Design review of the part built by this model. Coordinates are the model's own, in mm. A direction names the side the tool comes from. Give positions to 0.01 mm unless a question says otherwise; leave off trailing zeros. Write each loop counter-clockwise with the first axis right and the second up, starting at its lowest first coordinate (ties: lowest second). Pieces come first, ordered by that corner, then holes. Notation, with made-up numbers: (88, 23) -> (100, 23) arc R16 ccw to (100, 42) -> close; hole circle Ø4 at (33, 35). An arc over 180 degrees is marked (long way). Use CSV: the item, a comma, the result in double quotes.
```python
from build123d import *

# Parameters (mm, degrees)
SKETCH_1_W               = 60
SKETCH_1_H               = 10
EXTRUDE_1_DEPTH          = 8
SKETCH_2_W               = 10
SKETCH_2_H               = 21
SKETCH_2_R               = 3
EXTRUDE_2_DEPTH          = 5
FILLET_1_R               = 3
SKETCH_3_R               = 1.1
EXTRUDE_3_DEPTH          = 4
SKETCH_5_W               = 10
SKETCH_5_H               = 2
EXTRUDE_4_DEPTH          = 10
FILLET_4_R               = 1
SKETCH_4_R               = 1.6
CUT_EXTRUDE_1_DEPTH      = 17.792928464
CUT_EXTRUDE_1_DEPTH_BACK = 16.892331711


with BuildPart() as part:
    # 草图1 → 凸台-拉伸1 (new body)
    with BuildSketch(Plane(origin=(0, 0, 0), x_dir=(1, 0, 0), z_dir=(0, 1, 0))):
        Rectangle(SKETCH_1_W, SKETCH_1_H)
    extrude(amount=EXTRUDE_1_DEPTH)

    # 草图2 → 凸台-拉伸2 (add)
    with BuildSketch(Plane(origin=(30, 0, 0), x_dir=(0, 0, -1), z_dir=(1, 0, 0))):
        with Locations((0, -2.5)):
            Rectangle(SKETCH_2_W, SKETCH_2_H)
        with Locations((0, -8)):
            Circle(SKETCH_2_R, mode=Mode.SUBTRACT)
    extrude_2 = extrude(amount=-EXTRUDE_2_DEPTH)

    # 镜向1: 凸台-拉伸2 across plane
    add(extrude_2.mirror(Plane(origin=(0, 0, 0), x_dir=(0, 0, 1), z_dir=(1, 0, 0))))

    # 圆角1
    fillet_1_edges = [part.edges().sort_by_distance(p)[0] for p in [
        (27.5, -13, 5),
        (27.5, -13, -5),
        (-27.5, -13, -5),
        (-27.5, -13, 5),
    ]]
    fillet(fillet_1_edges, radius=FILLET_1_R)

    # 草图3 → 凸台-拉伸3 (add)
    with BuildSketch(Plane.ZY.offset(-5)):
        Polygon((-6.5, -2), (17.5, -2), (17.5, -8), (17.5, -10.376383694), (21.792928464, -10.376383694), (21.792928464, 2.519827065), (-10.892331711, 2.519827065), (-10.892331711, -10.376383694), (-6.5, -10.376383694), (-6.5, -8), align=None)
        with Locations((-8.5, -8)):
            Circle(SKETCH_3_R, mode=Mode.SUBTRACT)
        with Locations((19.5, -8)):
            Circle(SKETCH_3_R, mode=Mode.SUBTRACT)
    extrude(amount=-EXTRUDE_3_DEPTH)

    # 草图5 → 凸台-拉伸4 (add)
    with BuildSketch(Plane.ZY.offset(-5)):
        with Locations((0, -1)):
            Rectangle(SKETCH_5_W, SKETCH_5_H)
    extrude(amount=EXTRUDE_4_DEPTH)

    # 圆角4
    fillet_4_edges = [part.edges().sort_by_distance(p)[0] for p in [
        (5, 0.259913532, -5),
        (7, 2.519827065, -5),
        (9, 1.259913532, -5),
        (7, 2.519827065, -10.892331711),
        (5, 0.259913532, 5),
        (7, -10.376383694, -10.892331711),
        (7, 2.519827065, 5),
        (7, 2.519827065, 21.792928464),
        (7, -10.376383694, 21.792928464),
        (9, 1.259913532, 5),
        (9, 0, 0),
    ]]
    fillet(fillet_4_edges, radius=FILLET_4_R)

    # 草图4 → 切除-拉伸1 (cut, two sides)
    with BuildSketch(Plane.XY.offset(5)) as cut_extrude_1_sk:
        with Locations((-15, 4)):
            Circle(SKETCH_4_R)
        with Locations((15, 4)):
            Circle(SKETCH_4_R)
    extrude(amount=CUT_EXTRUDE_1_DEPTH, mode=Mode.SUBTRACT)
    extrude(cut_extrude_1_sk.sketch, amount=-CUT_EXTRUDE_1_DEPTH_BACK, mode=Mode.SUBTRACT)


solid = part.part
```
(1) Take a section at D-D (z = -8.5). Write out the cut boundary in (x, y), then the cut area to 3 significant figures.
Established:
outline,"(5, -10.38) -> (9, -10.38) -> (9, -9.1) -> (5, -9.1) -> close; (5, -6.9) -> (9, -6.9) -> (9, 2.52) -> (5, 2.52) -> close"
area,"42.8 mm2"
(2) Take a section at A-A (z = 0). Write out the cut boundary in (x, y).
Established:
outline,"(-30, -13) -> (-25, -13) -> (-25, -11) -> (-30, -11) -> close; (-30, -5) -> (-25, -5) -> (-25, 0) -> (-5, 0) -> (-5, -2) -> (9, -2) -> (9, -1) arc R1 cw to (10, 0) -> (25, 0) -> (25, -5) -> (30, -5) -> (30, 8) -> (-30, 8) -> close; (25, -13) -> (30, -13) -> (30, -11) -> (25, -11) -> close; hole circle Ø3.2 at (-15, 4); hole circle Ø3.2 at (15, 4)"
(3) Take a section at C-C (y = -8). State how many separate pieces and enclosed holes the cut face has, then the cut area to 3 significant figures.
Established:
separate pieces,"8"
enclosed holes,"0"
area,"57.1 mm2"
(4) Clearance check with flat-ended pins moving along their axes: pin 1 (3 mm diameter, centred on x = 6.5, z = -9, fed in from +Y); pin 2 (1 mm diameter, centred on x = 6.5, z = -8.5, fed in from -Y); pin 3 (3.5 mm diameter, centred on x = 15, y = 4, fed in from +Z); pin 4 (3 mm diameter, centred on x = -15, y = 4, fed in from +Z). State where each tip first meets the part, or that it passes through.
Established:
pin 1,"stops at y = 2.52"
pin 2,"stops at y = -10.38"
pin 3,"stops at z = 5"
pin 4,"passes through"
(5) Mouldability with a two-part tool opening along Y and no side actions: class faces 6 (the face through (-16.6, 4.07, 0.07)), 7 (the face through (27.46, -12.1, 4.14)), 8 (the face through (7, 2.52, -8)) as +Y half, -Y half, draft (parallel to the pull), parting line (faces both ways), or undercut.
Established:
face 6,"undercut"
face 7,"-Y half"
face 8,"+Y half"
(6) For line 1 along X through (y, z) = (-11.25, 2); line 2 along Y through (x, z) = (7.45, -8.5); line 3 along Y through (x, z) = (26, 0), list the stretches that pass through material, from the lowest coordinate up. Write a range as [from, to].
Established:
line 1,"x = [-30, -25], [25, 30]"
line 2,"y = [-10.38, -9.1], [-6.9, 2.52]"
line 3,"y = [-13, -11], [-5, 8]"
(7) Tool access review of faces 1 (the face through (-15, 0, 0)), 2 (the face through (30, -2, 0)), 3 (the face through (7, -6, -6.5)), 4 (the face through (4, -2, 3)), 5 (the face through (7, -4, 21.793)): name each direction out of +Z, -Z, +X, -X, +Y, -Y from which nothing blocks a thin tool from reaching the whole face with its end or side.
Established:
face 1,"+Z, -Z, -Y"
face 2,"+Z, -Z, +X, +Y, -Y"
face 3,"+X, -X, -Y"
face 4,"-Y"
face 5,"+Z, +X, -X, +Y, -Y"
(8) Take a section at B-B (x = 15). Write out the cut boundary in (y, z), then the cut area to 3 significant figures.
Established:
outline,"(0, -5) -> (2.4, -5) -> (2.4, 5) -> (0, 5) -> close; (5.6, -5) -> (8, -5) -> (8, 5) -> (5.6, 5) -> close"
area,"48.0 mm2"
